from build123d import *

# Parameters (mm, degrees)
F0_W     = 24
F0_H     = 7.9375
F1_DEPTH = 3.96875
F2_R     = 2.4
F3_DEPTH = 7.9385
F4_R     = 2.4
F5_DEPTH = 7.9385


with BuildPart() as f1:
    # F0 (on Top) → F1 (new body, symmetric)
    with BuildSketch(Plane.XY):
        Rectangle(F0_W, F0_H)
    extrude(amount=F1_DEPTH, both=True)

    # F2 (on face) → F3 (cut, through all)
    with BuildSketch(Plane.XZ.offset(3.96875)):
        Circle(F2_R)
        with Locations((8.8, 0)):
            Circle(F2_R)
        with Locations((-8.8, 0)):
            Circle(F2_R)
    extrude(amount=-F3_DEPTH, mode=Mode.SUBTRACT)

    # F4 (on face) → F5 (cut, through all)
    with BuildSketch(Plane.XY.offset(3.96875)):
        Circle(F4_R)
        with Locations((8.8, 0)):
            Circle(F4_R)
        with Locations((-8.8, 0)):
            Circle(F4_R)
    extrude(amount=-F5_DEPTH, mode=Mode.SUBTRACT)


solid = f1.part
CAD build for the part. Positions are in the model's coordinates, mm. Give positions to 0.01 mm unless a question says otherwise; leave off trailing zeros. Order: outer loops, then holes, each group sorted by start corner. A loop starts at its lowest first (then second) coordinate and runs counter-clockwise, first axis right, second up. Notation, with made-up numbers: (-27, -24) -> (-13, -24) arc R16 ccw to (-13, 2) -> close; hole circle Ø3 at (-7.5, 79.25). An arc over 180 degrees is marked (long way). Return JSON: item names as keys, results as strings.
Q1. Drill centre lines: line 1 (X direction, y = 1, z = -1); line 2 (Y direction, x = 8.8, z = 2.65); line 3 (X direction, y = -0.75, z = 0.25). Where is each one in solid material? Low to high.
Working result:
{"line 1": "-12 to -10.98, -6.62 to -2.18, 2.18 to 6.62, 10.98 to 12", "line 2": "-3.97 to -2.4, 2.4 to 3.97", "line 3": "-12 to -11.19, -6.41 to -2.39, 2.39 to 6.41, 11.19 to 12"}
Q2. Flat gauge pin, fed straight in: pin 1 (3 mm diameter, centred on x = 8.8, z = 0, fed in from +Y). Where does the tip first touch, or does it go through?
Working result:
{"pin 1": "through"}
Q3. Mould opens along Y. For faces 1 (the face through (0, 3.969, 3)), 2 (the face through (-1.905, -1.46, 2.453)), 3 (the face through (12, 0, 0)), 4 (the face through (6.895, -1.46, -2.398)) say: pulls with the +Y half, pulls with the -Y half, needs draft (parallel to the pull), parting line crosses it, or undercut.
Working result:
{"face 1": "pulls with the +Y half", "face 2": "undercut", "face 3": "needs draft", "face 4": "undercut"}
Q4. Saw through at A-A (x = 0). Write the cut outline in (y, z), then the cut area to 3 significant figures.
Working result:
{"outline": "(-3.97, -3.97) -> (-2.4, -3.97) -> (-2.4, -2.4) -> (-3.97, -2.4) -> close; (-3.97, 2.4) -> (-2.4, 2.4) -> (-2.4, 3.97) -> (-3.97, 3.97) -> close; (2.4, -3.97) -> (3.97, -3.97) -> (3.97, -2.4) -> (2.4, -2.4) -> close; (2.4, 2.4) -> (3.97, 2.4) -> (3.97, 3.97) -> (2.4, 3.97) -> close", "area": "9.84 mm²"}
Q5. Saw through at B-B (y = 3.75). Write the cut outline in (x, z).
Working result:
{"outline": "(-12, -3.97) -> (12, -3.97) -> (12, 3.97) -> (-12, 3.97) -> close; hole circle Ø4.8 at (-8.8, 0); hole circle Ø4.8 at (0, 0); hole circle Ø4.8 at (8.8, 0)"}
Q6. Saw through at D-D (y = 2). Write the cut outline in (x, z), then the cut area to 3 significant figures.
Working result:
{"outline": "(-12, -3.97) -> (-10.13, -3.97) -> (-10.13, -2) arc R2.4 cw to (-10.13, 2) -> (-10.13, 3.97) -> (-12, 3.97) -> close; (-7.47, -3.97) -> (-1.33, -3.97) -> (-1.33, -2) arc R2.4 cw to (-1.33, 2) -> (-1.33, 3.97) -> (-7.47, 3.97) -> (-7.47, 2) arc R2.4 cw to (-7.47, -2) -> close; (1.33, -3.97) -> (7.47, -3.97) -> (7.47, -2) arc R2.4 cw to (7.47, 2) -> (7.47, 3.97) -> (1.33, 3.97) -> (1.33, 2) arc R2.4 cw to (1.33, -2) -> close; (10.13, -3.97) -> (12, -3.97) -> (12, 3.97) -> (10.13, 3.97) -> (10.13, 2) arc R2.4 cw to (10.13, -2) -> close", "area": "109 mm²"}
